from build123d import *

# Parameters (mm, degrees)
CYLINDER044_R          = 1.55
CYLINDER044_DEPTH      = 10
CYLINDER042_R          = 3
CYLINDER042_DEPTH      = 10
CYLINDER043_R          = 3.5
CYLINDER043_DEPTH      = 1.6
BOX_W                  = 7
BOX_H                  = 11
BOX_DEPTH              = 1.6
BOX001_W               = 2
BOX001_H               = 21.6
BOX001_DEPTH           = 1.6
BOX001_PLACEMENT_ANGLE = 29.7
BOX002_W               = 2
BOX002_H               = 21.6
BOX002_DEPTH           = 1.6
BOX002_PLACEMENT_ANGLE = 29.7
BOX004_W               = 15
BOX004_H               = 4.55
BOX004_DEPTH           = 1.6
BOX003_W               = 11
BOX003_H               = 4
BOX003_DEPTH           = 1.6
CYLINDER040_W          = 11.75
CYLINDER040_H          = 1.6
CYLINDER040_ANGLE      = 180
CYLINDER039_W          = 15
CYLINDER039_H          = 1.6
CYLINDER039_ANGLE      = 180
FILLET006_R            = 1.2


with BuildPart() as cylinder044:
    # Cylinder044 → Cylinder044 (new body)
    with BuildSketch(Plane(origin=(0, 23, -0.5), x_dir=(1, 0, 0), z_dir=(0, 0, 1))):
        Circle(CYLINDER044_R)
    extrude(amount=CYLINDER044_DEPTH)


with BuildPart() as cylinder042:
    # Cylinder042 → Cylinder042 (new body)
    with BuildSketch(Plane(origin=(0, 23, -0.5), x_dir=(1, 0, 0), z_dir=(0, 0, 1))):
        Circle(CYLINDER042_R)
    extrude(amount=CYLINDER042_DEPTH)


with BuildPart() as cylinder043:
    # Cylinder043 → Cylinder043 (new body)
    with BuildSketch(Plane(origin=(0, 23, 0), x_dir=(1, 0, 0), z_dir=(0, 0, 1))):
        Circle(CYLINDER043_R)
    extrude(amount=CYLINDER043_DEPTH)


with BuildPart() as cube:
    # Box → Box (new body)
    with BuildSketch(Plane(origin=(-3.5, 12, 0), x_dir=(1, 0, 0), z_dir=(0, 0, 1))):
        with Locations((3.5, 5.5)):
            Rectangle(BOX_W, BOX_H)
    extrude(amount=BOX_DEPTH)


with BuildPart() as cube001:
    # Box001 → Box001 (new body)
    with BuildSketch(Plane.XY):
        with Locations((1, 10.8)):
            Rectangle(BOX001_W, BOX001_H)
    extrude(amount=BOX001_DEPTH)


with BuildPart() as cube001_1:
    # Box001 placement: moved
    add(cube001.part.moved(Location((12, 5, 0))).rotate(Axis((12, 5, 0), (0, 0, 1)), BOX001_PLACEMENT_ANGLE))


with BuildPart() as cube002:
    # Box002 → Box002 (new body)
    with BuildSketch(Plane.XY):
        with Locations((1, 10.8)):
            Rectangle(BOX002_W, BOX002_H)
    extrude(amount=BOX002_DEPTH)


with BuildPart() as cube002_1:
    # Box002 placement: moved
    add(cube002.part.moved(Location((12, 5, 0))).rotate(Axis((12, 5, 0), (0, 0, 1)), BOX002_PLACEMENT_ANGLE))


with BuildPart() as part_mirroring:
    # Part__Mirroring: instance of Cube002
    add(cube002_1.part.mirror(Plane(origin=(0, 0, 0), x_dir=(0, -1, 0), z_dir=(1, 0, 0))))


with BuildPart() as cube004:
    # Box004 → Box004 (new body)
    with BuildSketch(Plane(origin=(-7.5, 12, 0), x_dir=(1, 0, 0), z_dir=(0, 0, 1))):
        with Locations((7.5, 2.275)):
            Rectangle(BOX004_W, BOX004_H)
    extrude(amount=BOX004_DEPTH)


with BuildPart() as cube003:
    # Box003 → Box003 (new body)
    with BuildSketch(Plane(origin=(-5.5, 16, 0), x_dir=(1, 0, 0), z_dir=(0, 0, 1))):
        with Locations((5.5, 2)):
            Rectangle(BOX003_W, BOX003_H)
    extrude(amount=BOX003_DEPTH)


with BuildPart() as cylinder040:
    # Cylinder040 → Cylinder040 (revolve)
    with BuildSketch(Plane.XZ):
        with Locations((5.875, 0.8)):
            Rectangle(CYLINDER040_W, CYLINDER040_H)
    revolve(axis=Axis((0, 0, 0), (0, 0, 1)), revolution_arc=CYLINDER040_ANGLE)


with BuildPart() as fillet006:
    # Cylinder039 → Cylinder039 (revolve)
    with BuildSketch(Plane.XZ):
        with Locations((7.5, 0.8)):
            Rectangle(CYLINDER039_W, CYLINDER039_H)
    revolve(axis=Axis((0, 0, 0), (0, 0, 1)), revolution_arc=CYLINDER039_ANGLE)

    # Cut017: cut Cylinder040
    add(cylinder040.part, mode=Mode.SUBTRACT)

    # Fusion012: union Cylinder043, Cube, Cube001, Part__Mirroring, Cube004, Cube003
    add(cylinder043.part)
    add(cube.part)
    add(cube001_1.part)
    add(part_mirroring.part)
    add(cube004.part)
    add(cube003.part)

    # Fusion013: union Cylinder042
    add(cylinder042.part)

    # Cut018: cut Cylinder044
    add(cylinder044.part, mode=Mode.SUBTRACT)

    # Fillet006
    fillet006_edges = [fillet006.edges().sort_by_distance(p)[0] for p in [
        (-15, 0, 0.8),
        (-11.75, 0, 0.8),
        (11.75, 0, 0.8),
        (15, 0, 0.8),
    ]]
    fillet(fillet006_edges, radius=FILLET006_R)


with BuildPart() as fillet006_1:
    # Fillet006 placement: moved
    add(fillet006.part.moved(Location((0, 0, 2.25))))


solid = fillet006_1.part
Geometry: final body of the model. Coordinates: model frame, mm. A direction names the side the tool comes from. Round coordinates to 2 decimals unless told otherwise and drop trailing zeros. Order: outer loops, then holes, each group sorted by start corner. A loop starts at its lowest first (then second) coordinate and runs counter-clockwise, first axis right, second up. Notation, with made-up numbers: (-35.75, 87.25) -> (10.25, 87.25) arc R22 cw to (10.25, 120.25) -> close; hole circle Ø4 at (55, 39). An arc over 180 degrees is marked (long way). Put each result on its own line as item: value. Start each with the question number.
Q1. Line query: probe 1 along Z at (x, y) = (-11.25, 10.25); probe 2 along Y at (x, z) = (0, 6); probe 3 along X at (y, z) = (23.75, 4). Output: solid intervals per line, ascending.
Q2. Reachability of faces 1 (the cylindrical face through (-0.65, 20.07, 7.74)), 2 (the cylindrical face through (0.1, 26.5, 3)), 3 (the cylindrical face through (-12.1, 0.3, 3.1)) from +Z, -Z, +X, -X, +Y, -Y: full face, straight path, thin tool, end or side. Return the list, or none.
Q3. First-contact query: pin 1 (1 mm diameter, centred on y = 14.5, z = 4, fed in from -X); pin 2 (4 mm diameter, centred on x = 10.5, z = 6.5, fed in from -Y); pin 3 (5 mm diameter, centred on x = 0, y = 23, fed in from +Z); pin 4 (5 mm diameter, centred on x = 2, z = 9.5, fed in from +Y). Flat tips, straight axial feed; report the tip coordinate or a pass-through.
Q4. Section C-C on y = 10.5. Return the cut outline in (x, z), and give its area (3 significant figures).
Q5. Pull-direction query (X, two-part tool) for faces 4 (the flat face through (7.63, 16.7, 3.04)), 5 (the cylindrical face through (-0.65, 20.07, 2)), 6 (the cylindrical face through (12.1, 0.3, 3.1)); classes: +X half, -X half, draft (parallel to the pull), parting line (faces both ways), or undercut.
Q6. Section D-D on y = 23. Return the cut outline in (x, z), and give its area (3 significant figures).
Q7. Section A-A on x = 0. Return the cut outline in (y, z), and give its area (3 significant figures).
Ans:
1. probe 1: z = 2.25 to 3.85
1. probe 2: y = 20 to 21.45, 24.55 to 26
1. probe 3: x = -2.9 to -1.36, 1.36 to 2.9
2. face 1: +Z
2. face 2: +Z, -Z, +Y
2. face 3: +Z, -Z, -Y
3. pin 1: stops at x = -9.16
3. pin 2: passes through
3. pin 3: stops at z = 11.75
3. pin 4: stops at y = 26
4. outline: (-11.17, 2.25) -> (-5.27, 2.25) -> (-5.27, 3.85) -> (-11.17, 3.85) -> close; (5.27, 2.25) -> (11.17, 2.25) -> (11.17, 3.85) -> (5.27, 3.85) -> close
4. area: 18.9 mm2
5. face 4: +X half
5. face 5: parting line
5. face 6: undercut
6. outline: (-4.04, 2.25) -> (-3, 2.25) -> (-3, 1.75) -> (-1.55, 1.75) -> (-1.55, 11.75) -> (-3, 11.75) -> (-3, 3.85) -> (-4.04, 3.85) -> close; (1.55, 1.75) -> (3, 1.75) -> (3, 2.25) -> (4.04, 2.25) -> (4.04, 3.85) -> (3, 3.85) -> (3, 11.75) -> (1.55, 11.75) -> close
6. area: 32.3 mm2
7. outline: (11.75, 2.25) -> (20, 2.25) -> (20, 1.75) -> (21.45, 1.75) -> (21.45, 11.75) -> (20, 11.75) -> (20, 3.85) -> (11.75, 3.85) -> close; (24.55, 1.75) -> (26, 1.75) -> (26, 2.25) -> (26.5, 2.25) -> (26.5, 3.85) -> (26, 3.85) -> (26, 11.75) -> (24.55, 11.75) -> close
7. area: 43.0 mm2
